Check sheet for the modelled part. Datum: model origin and axes. Units: mm. A direction names the side the tool comes from. Give positions to 0.01 mm unless a question says otherwise; leave off trailing zeros. Order: outer loops, then holes, each group sorted by start corner. A loop starts at its lowest first (then second) coordinate and runs counter-clockwise, first axis right, second up.
Autodesk Inventor part; units mm, degrees
ref_plane "YZ Plane" through (0, 0, 0) normal (1, 0, 0) x (0, 1, 0)
ref_plane "XZ Plane" through (0, 0, 0) normal (0, 1, 0) x (-1, 0, 0)
ref_plane "XY Plane" through (0, 0, 0) normal (0, 0, 1) x (1, 0, 0)
sketch "Sketch1" plane through (0, 0, 0) normal (0, 1, 0) x (-1, 0, 0)
  line L0 (0, 0) -> (361.1993, 0) construction
  line L1 (361.1993, 0) -> (361.1993, -361.1993) construction
  line L2 (361.1993, -361.1993) -> (0, -361.1993) construction
  line L3 (0, -361.1993) -> (0, 0) construction
sketch "Sketch2" plane through (0, 0, 0) normal (0, 1, 0) x (-1, 0, 0)
  line L0 (0, -180.5996) -> (11.43, -180.5996)
  line L1 (11.43, -180.5996) -> (180.5997, -72.009)
  line L2 (180.5997, -289.1903) -> (11.43, -180.5996)
  line L3 (361.1993, -180.5996) -> (349.7693, -180.5996)
  line L4 (349.7693, -180.5996) -> (180.5997, -72.009)
  line L5 (180.5997, -289.1903) -> (349.7693, -180.5996)
  line L6 (115.508, -119.0216) -> (145.1807, -119.0216)
  line L7 (145.1807, -119.0216) -> (145.1807, -242.5337)
  line L8 (145.1807, -242.5337) -> (115.508, -242.5337)
  line L9 (115.508, -242.5337) -> (115.508, -119.0216)
  line L10 (165.8332, -118.9647) -> (165.8332, -242.4769)
  line L11 (165.8332, -242.4769) -> (195.5355, -242.4769)
  line L12 (195.5355, -242.4769) -> (195.5355, -195.5556)
  line L13 (195.5355, -195.5556) -> (225.8549, -195.5556)
  line L14 (225.8549, -195.5556) -> (236.0754, -180.9592)
  line L15 (236.0754, -180.9592) -> (225.5562, -165.8753)
  line L16 (225.5562, -165.8753) -> (195.5355, -165.8753)
  line L17 (195.5355, -165.8753) -> (195.5355, -148.6741)
  line L18 (195.5355, -148.6741) -> (225.5562, -148.6741)
  line L19 (225.5562, -148.6741) -> (235.7293, -133.6668)
  line L20 (235.7293, -133.6668) -> (225.8549, -118.9647)
  line L21 (225.8549, -118.9647) -> (165.8332, -118.9647)
  line L22 (236.3576, -118.9647) -> (246.1353, -118.9647)
  line L23 (246.1353, -118.9647) -> (256.2661, -133.6668)
  line L24 (236.0628, -148.731) -> (246.0969, -148.731)
  line L25 (246.0969, -148.731) -> (256.2661, -133.6668)
  line L26 (236.3576, -118.9647) -> (246.2319, -133.6668)
  line L27 (236.0628, -148.731) -> (246.2319, -133.6668)
  line L28 (236.3576, -165.8976) -> (246.1353, -165.8976)
  line L29 (246.1353, -165.8976) -> (256.2661, -180.5996)
  line L30 (236.0628, -195.6639) -> (246.0969, -195.6639)
  line L31 (246.0969, -195.6639) -> (256.2661, -180.5996)
  line L32 (236.3576, -165.8976) -> (246.2319, -180.5996)
  line L33 (236.0628, -195.6639) -> (246.2319, -180.5996)
  point P0 (0, 0)
  dimension "d1" = 11.43
  dimension "d3" = 11.43
  dimension "d4" = 125
  dimension "d5" = 90
extrude "Extrusion1" add sketch "Sketch2" along normal blind 38.1
properties part number "TeamIF"
(1) Release check for a two-part mould opening along X. For faces 1 (the face through (-205, 38.1, -204)), 2 (the face through (-266.369, 18.783, -127.064)), 3 (the face through (-130, 19, -119.022)) record: released by +X, released by -X, zero draft, split by the parting line, or undercut.
Response values:
face 1: zero draft
face 2: released by -X
face 3: undercut
(2) Cross-section at A-A on x = -219. Enter the section's corners in (y, z), then the cut area to 3 significant figures.
Response values:
outline: (0, -264.54) - (38.1, -264.54) - (38.1, -195.56) - (0, -195.56) - close; (0, -165.88) - (38.1, -165.88) - (38.1, -148.67) - (0, -148.67) - close; (0, -118.96) - (38.1, -118.96) - (38.1, -96.66) - (0, -96.66) - close
area: 4,130 mm2
(3) Material ranges on L1, parallel to Z at x = -244.5, y = 34.5; L2, parallel to X at y = 21.5, z = -235; L3, parallel to Z at x = -244, y = 7.5, recorded low to high.
Response values:
L1: z = -248.17 to -195.66, -183.17 to -178.02, -165.9 to -148.73, -136.23 to -131.09, -118.96 to -113.03
L2: x = -265.02 to -195.54, -165.83 to -145.18, -115.51 to -96.18
L3: z = -248.49 to -195.66, -183.91 to -177.28, -165.9 to -148.73, -136.97 to -130.34, -118.96 to -112.71
(4) Gauge pin test, flat ends, axial feed: pin 1 Ø11.5 at (y, z) = (25.5, -222.5) entering from +X; pin 2 Ø8 at (x, y) = (-240, 24) entering from +Z; pin 3 Ø9 at (x, y) = (-126.5, 25) entering from +Z. Record the tip position at first contact, or that the pin passes through.
Response values:
pin 1: stops at x = -67.75
pin 2: stops at z = -107.57
pin 3: stops at z = -103.85
(5) Cross-section at D-D on x = -130.5. Enter the section's corners in (y, z).
Response values:
outline: (0, -257.03) - (38.1, -257.03) - (38.1, -242.53) - (0, -242.53) - close; (0, -119.02) - (38.1, -119.02) - (38.1, -104.17) - (0, -104.17) - close
(6) Set-up check for faces 4 (the face through (-97.199, 18.783, -235.655)), 5 (the face through (-230.894, 18.783, -188.36)): record each of +Z, -Z, +X, -X, +Y, -Y from which the full face is reachable in a straight line by a thin tool's end or side.
Response values:
face 4: -Z, +X, +Y, -Y
face 5: +Y, -Y
(7) Cross-section at C-C on y = 29. Count the separate pieces of the cut face and the enclosed holes in it, then the cut area to 3 significant figures.
Response values:
separate pieces: 1
enclosed holes: 4
area: 26,700 mm2
(8) Cross-section at B-B on z = -233.5. Enter the section's corners in (x, y), then the cut area to 3 significant figures.
Response values:
outline: (-267.36, 0) - (-195.54, 0) - (-195.54, 38.1) - (-267.36, 38.1) - close; (-165.83, 0) - (-145.18, 0) - (-145.18, 38.1) - (-165.83, 38.1) - close; (-115.51, 0) - (-93.84, 0) - (-93.84, 38.1) - (-115.51, 38.1) - close
area: 4,350 mm2
